Design review of the part shown in the three views and the two pictorial views. Dimensions are in mm from the part's minimum x, y and z. Round coordinates to 2 decimals unless told otherwise and drop trailing zeros. Order: outer loops, then holes, each group sorted by start corner. A loop starts at its lowest first (then second) coordinate and runs counter-clockwise, first axis right, second up. Notation, with made-up numbers: (-5, 29.5) -> (44, 29.5) arc R22 ccw to (44, 42.5) -> close; hole circle Ø6 at (-34, 7.25). An arc over 180 degrees is marked (long way). Put each result on its own line as item: value. Start each with the question number.
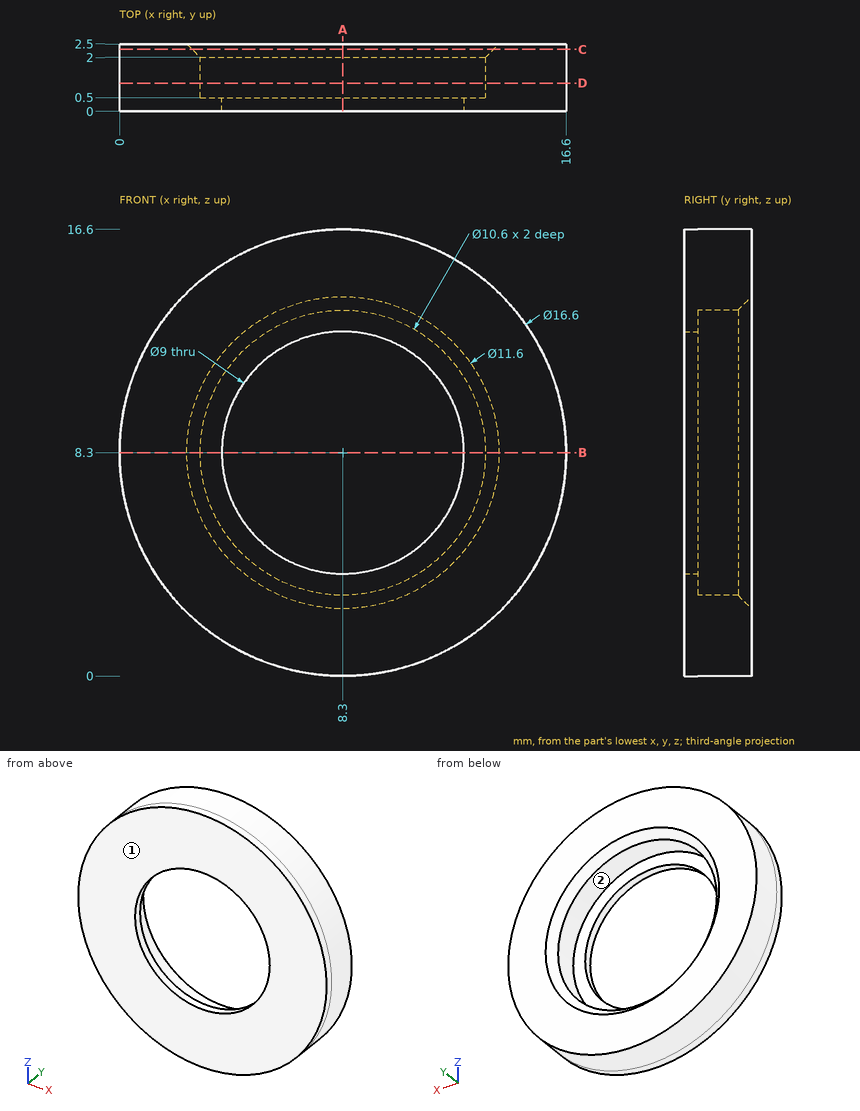
Q1. Take a section at C-C on y = 2.3. Give the boundary of the cut face in (x, z).
Q2. Clearance check with flat-ended pins moving along their axes: pin 1 Ø1.5 at (x, y) = (9.5, 2) entering from +Z; pin 2 Ø1 at (y, z) = (0.5, 2) entering from +X. State where each tip first meets the part, or that it passes through.
Q3. Take a section at A-A on x = 8.3. Give the boundary of the cut face in (y, z).
Q4. Take a section at D-D on y = 1.05. Give the boundary of the cut face in (x, z), and give its area (3 significant figures).
Q5. Draft analysis for pull direction Z (two halves, no side actions). For the marked faces 1 and 2, state which applies: +Z half, -Z half, draft (parallel to the pull), parting line (faces both ways), or undercut.
Q6. Take a section at B-B on z = 8.3. Give the boundary of the cut face in (x, y).
Q7. Wall thickness on probe 1 along Z at (x, y) = (8.25, 0.55); probe 2 along X at (y, z) = (0.3, 8.25); probe 3 along Z at (x, y) = (5, 0.3): over which ranges is each line inside the solid? List them lowest first. Write a range as [from, to].
Calculated:
1. outline: circle Ø16.6 at (8.3, 8.3); hole circle Ø11.2 at (8.3, 8.3)
2. pin 1: stops at z = 16.59
2. pin 2: stops at x = 14.24
3. outline: (0, 0) -> (2.5, 0) -> (2.5, 2.5) -> (2, 3) -> (0.5, 3) -> (0.5, 3.8) -> (0, 3.8) -> close; (0, 12.8) -> (0.5, 12.8) -> (0.5, 13.6) -> (2, 13.6) -> (2.5, 14.1) -> (2.5, 16.6) -> (0, 16.6) -> close
4. outline: circle Ø16.6 at (8.3, 8.3); hole circle Ø10.6 at (8.3, 8.3)
4. area: 128 mm²
5. face 1: draft
5. face 2: undercut
6. outline: (0, 0) -> (3.8, 0) -> (3.8, 0.5) -> (3, 0.5) -> (3, 2) -> (2.5, 2.5) -> (0, 2.5) -> close; (12.8, 0) -> (16.6, 0) -> (16.6, 2.5) -> (14.1, 2.5) -> (13.6, 2) -> (13.6, 0.5) -> (12.8, 0.5) -> close
7. probe 1: z = [0, 3], [13.6, 16.6]
7. probe 2: x = [0, 3.8], [12.8, 16.6]
7. probe 3: z = [0.68, 5.24], [11.36, 15.92]
